Autodesk Inventor part; units mm, degrees
ref_plane "YZ Plane" through (0, 0, 0) normal (1, 0, 0) x (0, 1, 0)
ref_plane "XZ Plane" through (0, 0, 0) normal (0, 1, 0) x (-1, 0, 0)
ref_plane "XY Plane" through (0, 0, 0) normal (0, 0, 1) x (1, 0, 0)
sketch "Sketch1" plane through (0, 0, 0) normal (1, 0, 0) x (0, 1, 0)
  line L0 (0, 25.9556) -> (0, 21.9556)
  line L1 (0, 21.9556) -> (15, 21.9556)
  line L2 (15, 21.9556) -> (15, -12.0444)
  line L3 (15, -12.0444) -> (0, -12.0444)
  line L4 (0, -12.0444) -> (0, -16.0444)
  line L5 (0, -16.0444) -> (19, -16.0444)
  line L6 (19, -16.0444) -> (19, 25.9556)
  line L7 (19, 25.9556) -> (0, 25.9556)
  point P0 (0, 0)
  dimension "d0" = 4
  dimension "d1" = 4
  dimension "d2" = 15
  dimension "d3" = 42
extrude "Extrusion1" add sketch "Sketch1" along normal blind 50
sketch "Sketch2" plane through (0, 0, 25.9556) normal (0, 0, 1) x (1, 0, 0)
  line L0 (50, 0) -> (25, 0)
  line L1 (25, 0) -> (25, 15)
  line L2 (25, 15) -> (50, 15)
  line L3 (50, 15) -> (50, 0)
  point P0 (0, 0)
  dimension "d6" = 15
  dimension "d7" = 25
extrude "Extrusion2" cut sketch "Sketch2" against normal blind 50
fillet "Fillet1" radius 21 2 edges at (50, 17, 25.9556) (50, 17, -16.0444)
hole "Hole1" at (29, 19, 4.9556) direction (0, -1, 0) diameter 15 depth 8 tip angle 118
hole "Hole2" at (29, 19, -6.0444) direction (0, -1, 0) diameter 2 depth 8 tip angle 118
hole "Hole6" at (6, 8, -16.0444) direction (0, 0, 1) diameter 4 depth 42
pattern_circular "Circular Pattern1" count 4 over 360 about axis through (29, 15, 4.9556) along (0, 1, 0) of "Hole2"
sketch "Sketch3" plane through (0, 0, 25.9556) normal (0, 0, 1) x (1, 0, 0)
  line L0 (25, 15) -> (25, 0)
  line L1 (0, 19) -> (29, 19)
  line L2 (25, 0) -> (21, 0)
  line L3 (21, 0) -> (21, 19)
  line L4 (21, 19) -> (25, 19)
  line L5 (25, 19) -> (25, 0)
  point P0 (0, 0)
  dimension "d68" = 4
extrude "Extrusion3" add sketch "Sketch3" along normal blind 4
sketch "Sketch4" plane through (0, 0, -16.0444) normal (0, 0, -1) x (-1, 0, 0)
  line L0 (0, 0) -> (-25, 0)
  line L1 (0, 19) -> (-21, 19)
  line L2 (-25, 0) -> (-21, 0)
  line L3 (-21, 0) -> (-21, 19)
  line L4 (-21, 19) -> (-25, 19)
  line L5 (-25, 19) -> (-25, 0)
  dimension "d73" = 4
extrude "Extrusion4" add sketch "Sketch4" along normal blind 4
properties part number "BaseJointMotorMount"
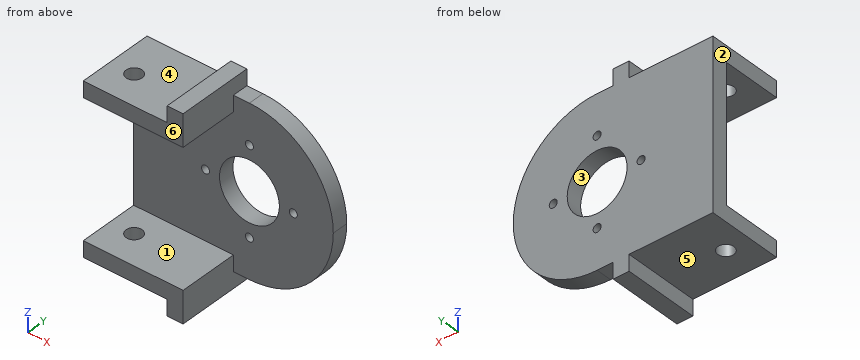
The model under review builds one solid part; all positions refer to its coordinate system, in mm. Face numbers are marked on the shaded views. A direction names the side the tool comes from. Coordinates: 2 decimals unless noted, no trailing zeros. Loops run counter-clockwise (first coordinate to the right, second up) from the corner with the lowest first, then second, coordinate; pieces in that order, holes last. Notation, with made-up numbers: (22, -3.75) -> (76, -3.75) arc R9 cw to (76, 11.25) -> close; hole circle Ø10 at (9.5, 21.25). An arc over 180 degrees is marked (long way). Use a Markdown table: item, result. Add a question column.
1. Clearance check with flat-ended pins moving along their axes: pin 1 Ø12 at (x, z) = (30, -3) entering from -Y; pin 2 Ø1.2 at (x, y) = (26.5, 17.5) entering from +Z; pin 3 Ø2 at (x, y) = (7, 13) entering from -Z. State where each tip first meets the part, or that it passes through.
2. Add section C-C on y = 11.5. Write out the cut boundary in (x, z), plus the area to 3 significant figures.
3. To check wall thickness, follow line 1 (Z direction, x = 19.5, y = 1.5); line 2 (Z direction, x = 24.5, y = 10.75); line 3 (Y direction, x = 42, z = 12.5). State the ranges of each line that lie inside material, in increasing order.
4. Add section A-A on y = 8. Write out the cut boundary in (x, z).
5. Add section B-B on x = 18. Write out the cut boundary in (y, z).
6. Add section D-D on x = 6. Write out the cut boundary in (y, z).
7. Draft analysis for pull direction Z (two halves, no side actions). For the marked faces 3, 4, 5 and 6, state which applies: pulls with the +Z half, pulls with the -Z half, needs draft (parallel to the pull), parting line crosses it, or undercut.
8. Machinability: for the marked faces 1 and 2, which of the approach directions +Z, -Z, +X, -X, +Y, -Y give a long, thin tool a straight path to every point of the face, cutting with its end or side? Answer none if there is none.
Returned:
| question | item | result |
|---|---|---|
| 1 | pin 1 | stops at y = 15 |
| 1 | pin 2 | stops at z = 25.96 |
| 1 | pin 3 | stops at z = -16.04 |
| 2 | outline | (0, -16.04) -> (21, -16.04) -> (21, -20.04) -> (25, -20.04) -> (25, -12.04) -> (0, -12.04) -> close; (0, 21.96) -> (25, 21.96) -> (25, 29.96) -> (21, 29.96) -> (21, 25.96) -> (0, 25.96) -> close |
| 2 | area | 232 mm² |
| 3 | line 1 | z = -16.04 to -12.04, 21.96 to 25.96 |
| 3 | line 2 | z = -20.04 to -12.04, 21.96 to 29.96 |
| 3 | line 3 | y = 15 to 19 |
| 4 | outline | (0, -16.04) -> (4, -16.04) -> (4, -12.04) -> (0, -12.04) -> close; (0, 21.96) -> (4, 21.96) -> (4, 25.96) -> (0, 25.96) -> close; (8, -16.04) -> (21, -16.04) -> (21, -20.04) -> (25, -20.04) -> (25, -12.04) -> (8, -12.04) -> close; (8, 21.96) -> (25, 21.96) -> (25, 29.96) -> (21, 29.96) -> (21, 25.96) -> (8, 25.96) -> close |
| 5 | outline | (0, -16.04) -> (19, -16.04) -> (19, 3.96) -> (15, 3.96) -> (15, -12.04) -> (0, -12.04) -> close; (0, 21.96) -> (15, 21.96) -> (15, 5.96) -> (19, 5.96) -> (19, 25.96) -> (0, 25.96) -> close |
| 6 | outline | (0, -16.04) -> (6, -16.04) -> (6, -12.04) -> (0, -12.04) -> close; (0, 21.96) -> (6, 21.96) -> (6, 25.96) -> (0, 25.96) -> close; (10, -16.04) -> (19, -16.04) -> (19, 25.96) -> (10, 25.96) -> (10, 21.96) -> (15, 21.96) -> (15, -12.04) -> (10, -12.04) -> close |
| 7 | face 3 | undercut |
| 7 | face 4 | pulls with the +Z half |
| 7 | face 5 | pulls with the -Z half |
| 7 | face 6 | needs draft |
| 8 | face 1 | +X, -X, -Y |
| 8 | face 2 | +Z, -Z, -X, +Y, -Y |
